Geometry: see drawing. Coordinates: mm, zero at the bounding-box minimum. A direction names the side the tool comes from. Coordinates: 2 decimals unless noted, no trailing zeros. Loops run counter-clockwise (first coordinate to the right, second up) from the corner with the lowest first, then second, coordinate; pieces in that order, holes last. Notation, with made-up numbers: (42, 43) - (80, 43) arc R13 ccw to (80, 50) - close; hole circle Ø8 at (-9.75, 88.5). An arc over 180 degrees is marked (long way). Use one line per item in the form item = value.
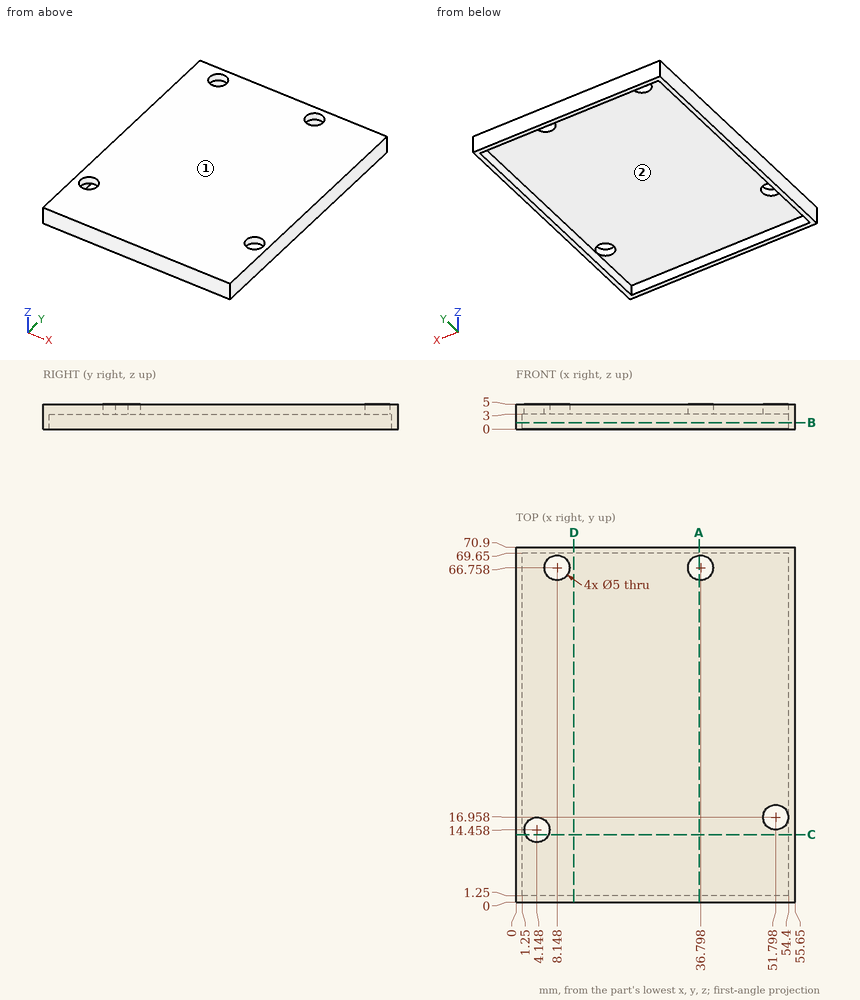
Q1. Cut plane C-C, the plane y = 13.5. Return loops of the section in (x, z).
Check values:
outline = (0, 0) - (1.25, 0) - (1.25, 3) - (1.84, 3) - (1.84, 5) - (0, 5) - close; (6.46, 3) - (54.4, 3) - (54.4, 0) - (55.65, 0) - (55.65, 5) - (6.46, 5) - close
Q2. Cut plane A-A, the plane x = 36.5. Return loops of the section in (y, z).
Check values:
outline = (0, 0) - (1.25, 0) - (1.25, 3) - (64.28, 3) - (64.28, 5) - (0, 5) - close; (69.24, 3) - (69.65, 3) - (69.65, 0) - (70.9, 0) - (70.9, 5) - (69.24, 5) - close
Q3. Ray query, line 1 along Y through (x, z) = (3, 1.5); line 2 along X through (y, z) = (34, 0.45); line 3 along Z through (x, y) = (17.5, 29.5). Return the intervals inside material, ascending. Write a range as [from, to].
Check values:
line_1 = [0, 1.25], [69.65, 70.9]
line_2 = [0, 1.25], [54.4, 55.65]
line_3 = [3, 5]
Q4. Cut plane D-D, the plane x = 11.5. Return loops of the section in (y, z).
Check values:
outline = (0, 0) - (1.25, 0) - (1.25, 3) - (69.65, 3) - (69.65, 0) - (70.9, 0) - (70.9, 5) - (0, 5) - close
Q5. Cut plane B-B, the plane z = 1.3. Return loops of the section in (x, y).
Check values:
outline = (0, 0) - (55.65, 0) - (55.65, 70.9) - (0, 70.9) - close; hole (1.25, 1.25) - (54.4, 1.25) - (54.4, 69.65) - (1.25, 69.65) - close
Q6. First-contact query: P1, Ø16, axis at x = 38.5, y = 50, coming from the -Z side; P2, Ø4, axis at x = 36.8, y = 66.76, coming from the +Z side. Flat tips, straight axial feed; report the tip coordinate or a pass-through.
Check values:
P1 = 3
P2 = through
Q7. Set-up query: the marked faces 1 and 2. Return all of +Z, -Z, +X, -X, +Y, -Y with unobstructed straight access to the full face (end or side cutting, diameter ignored); none if empty.
Check values:
face_1 = +Z, +X, -X, +Y, -Y
face_2 = -Z
